Here's the drawing with two shaded views (mm, measured from the low corner). I have some questions. A direction names the side the tool comes from. Coordinates: 2 decimals unless noted, no trailing zeros. Write each loop counter-clockwise with the first axis right and the second up, starting at its lowest first coordinate (ties: lowest second). Pieces come first, ordered by that corner, then holes.
Item 1: If we section it at B-B (z = 25): Please give me the cut outline in (x, y).
Item 2: I'm going to push flat-ended pins straight in: pin 1 Ø5 at (y, z) = (12.5, 32) entering from +X; pin 2 Ø4 at (x, y) = (10, 2.5) entering from +Z. Where does each tip first touch, or does it pass through?
Item 3: If I drill on line 1 (Y direction, x = 28, z = 1.4); line 2 (X direction, y = 17, z = 22.5); line 3 (Z direction, x = 54.6, y = 12.5), over which ranges is the centre line in solid material (lowest first)?
Item 4: If we section it at D-D (z = 29.5): Please give me the cut outline in (x, y).
Item 5: We'd pull the mould along X, two halves only. Please class the marked faces 1, 2 and 3: +X half, -X half, draft (parallel to the pull), parting line (faces both ways), or undercut.
Item 6: If we section it at C-C (y = 19.5): Please give me the cut outline in (x, z).
Item 7: For the marked faces 4 and 5, which set-ups out of +Z, -Z, +X, -X, +Y, -Y let a thin tool reach every point of the face, with its end or its side?
Item 8: If we section it at A-A (x = 9.4): Please give me the cut outline in (y, z).
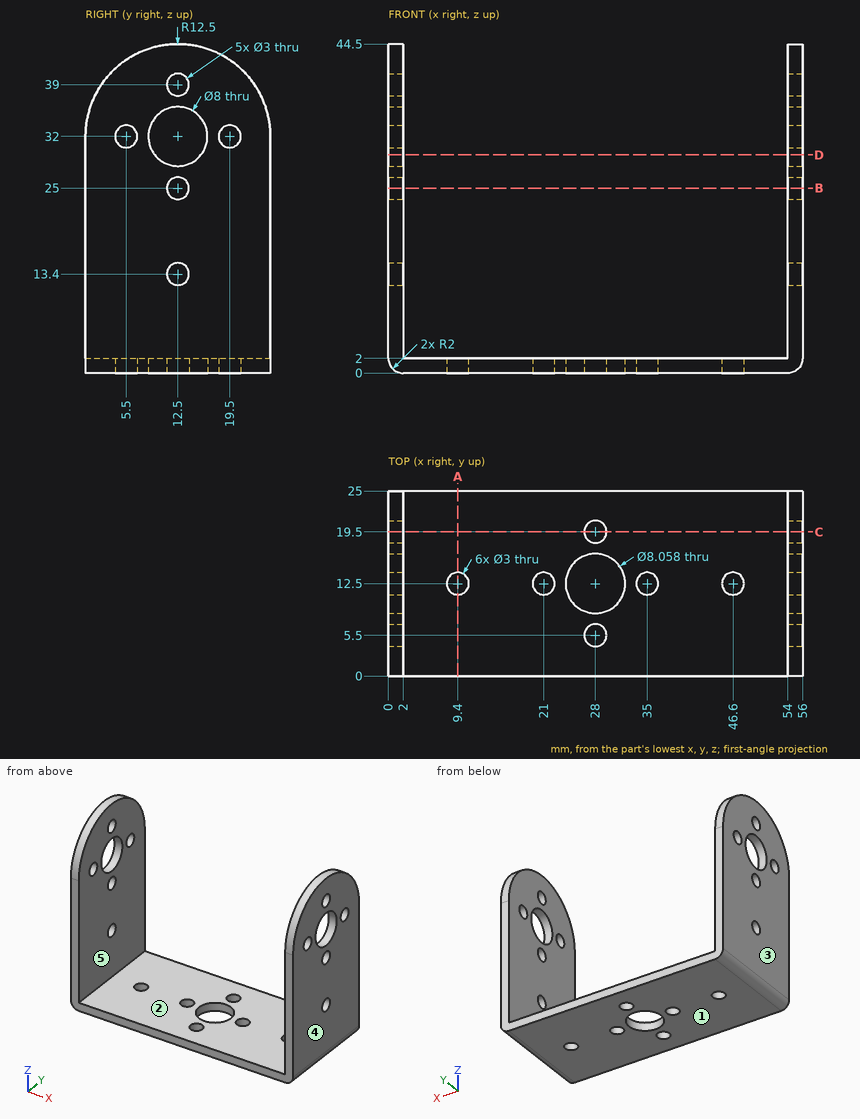
Answer list:
1. outline: (0, 0) - (2, 0) - (2, 11) - (0, 11) - close; (0, 14) - (2, 14) - (2, 25) - (0, 25) - close; (54, 0) - (56, 0) - (56, 11) - (54, 11) - close; (54, 14) - (56, 14) - (56, 25) - (54, 25) - close
2. pin 1: passes through
2. pin 2: stops at z = 2
3. line 1: y = 0 to 4, 7 to 8.47, 16.53 to 18, 21 to 25
3. line 2: x = 0 to 2, 54 to 56
3. line 3: z = 0.09 to 11.9, 14.9 to 23.5, 26.5 to 28, 36 to 37.5, 40.5 to 44.5
4. outline: (0, 0) - (2, 0) - (2, 9.38) - (0, 9.38) - close; (0, 15.62) - (2, 15.62) - (2, 25) - (0, 25) - close; (54, 0) - (56, 0) - (56, 9.38) - (54, 9.38) - close; (54, 15.62) - (56, 15.62) - (56, 25) - (54, 25) - close
5. face 1: draft
5. face 2: undercut
5. face 3: -X half
6. outline: (0, 2) arc R2 ccw to (2, 0) - (26.5, 0) - (26.5, 2) - (2, 2) - (2, 30.5) - (0, 30.5) - close; (0, 33.5) - (2, 33.5) - (2, 42.36) - (0, 42.36) - close; (29.5, 0) - (54, 0) arc R2 ccw to (56, 2) - (56, 30.5) - (54, 30.5) - (54, 2) - (29.5, 2) - close; (54, 33.5) - (56, 33.5) - (56, 42.36) - (54, 42.36) - close
7. face 4: +Z, -Z, +X, +Y, -Y
7. face 5: +Z, +Y, -Y
8. outline: (0, 0) - (11, 0) - (11, 2) - (0, 2) - close; (14, 0) - (25, 0) - (25, 2) - (14, 2) - close
